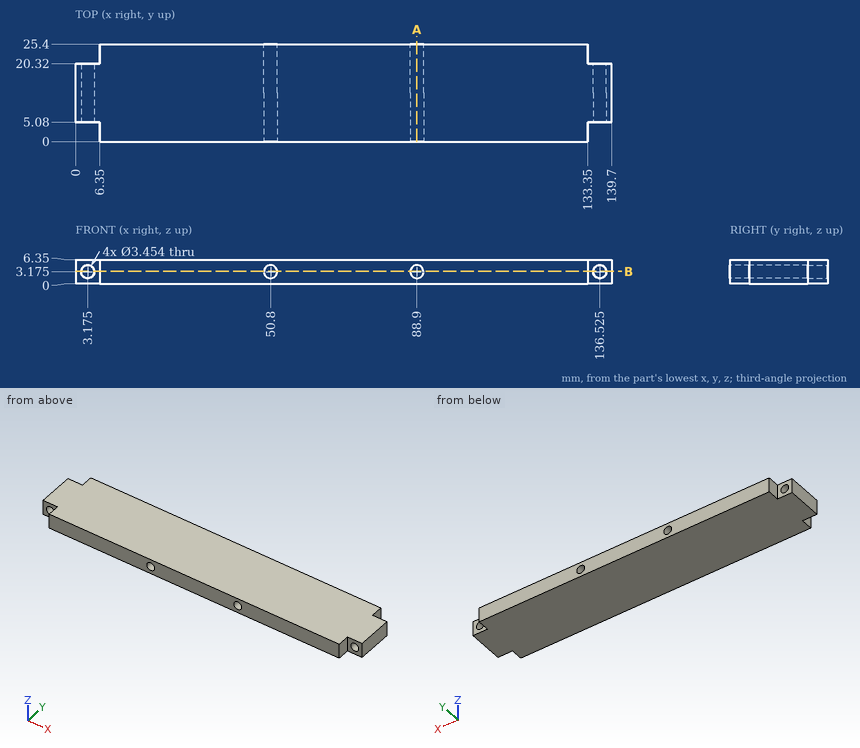
Geometry: see drawing. Coordinates: mm, zero at the bounding-box minimum. Give positions to 0.01 mm unless a question says otherwise; leave off trailing zeros. Loops run counter-clockwise (first coordinate to the right, second up) from the corner with the lowest first, then second, coordinate; pieces in that order, holes last. Notation, with made-up numbers: (66.5, 73.25) -> (99.5, 73.25) arc R30 ccw to (99.5, 102.25) -> close; hole circle Ø10 at (18.5, 20.5). An arc over 180 degrees is marked (long way). Answer as a JSON object with one key per item and string values. Group by question number.
Item 1: Line query: probe 1 along X at (y, z) = (3.5, 3); probe 2 along Z at (x, y) = (50.8, 7.5); probe 3 along X at (y, z) = (5.5, 4.75) (1 decimal). Output: solid intervals per line, ascending.
Item 2: Cut plane B-B, the plane z = 3.25. State how many separate pieces and enclosed holes the cut face has, and give its area (3 significant figures).
Item 3: Pin query (flat end, axial travel): P1, Ø3, axis at x = 28.5, y = 3.5, coming from the -Z side; P2, Ø3, axis at x = 50.8, z = 3.175, coming from the +Y side; P3, Ø1.5, axis at y = 23, z = 4, coming from the +X side; P4, Ø1.9, axis at x = 137.5, z = 4, coming from the +Y side. Return the tip coordinate at first contact, or that it passes through.
Item 4: Cut plane A-A, the plane x = 88.9. Return the cut outline in (y, z).
Checks:
{
 "1": {"probe 1": "x = 6.35 to 49.08, 52.52 to 87.18, 90.62 to 133.35", "probe 2": "z = 0 to 1.45, 4.9 to 6.35", "probe 3": "x = 0 to 2.5, 3.9 to 50.1, 51.5 to 88.2, 89.6 to 135.8, 137.2 to 139.7"},
 "2": {"separate pieces": "5", "enclosed holes": "0", "area": "3,140 mm²"},
 "3": {"P1": "stops at z = 0", "P2": "passes through", "P3": "stops at x = 133.35", "P4": "stops at y = 20.32"},
 "4": {"outline": "(0, 0) -> (25.4, 0) -> (25.4, 1.45) -> (0, 1.45) -> close; (0, 4.9) -> (25.4, 4.9) -> (25.4, 6.35) -> (0, 6.35) -> close"}
}
